Answer from the drawing. Dimensions are ordinates in mm from the lowest x, y and z of the part. Coordinates: 2 decimals unless noted, no trailing zeros. Order: outer loops, then holes, each group sorted by start corner. A loop starts at its lowest first (then second) coordinate and runs counter-clockwise, first axis right, second up. Notation, with made-up numbers: M 58.25,-29.75 L 81.25,-29.75 A15 cw 81.25,-10.75 Z; hole C -18,89.5 d2. An arc over 180 degrees is marked long. Use a Markdown table: item, result.
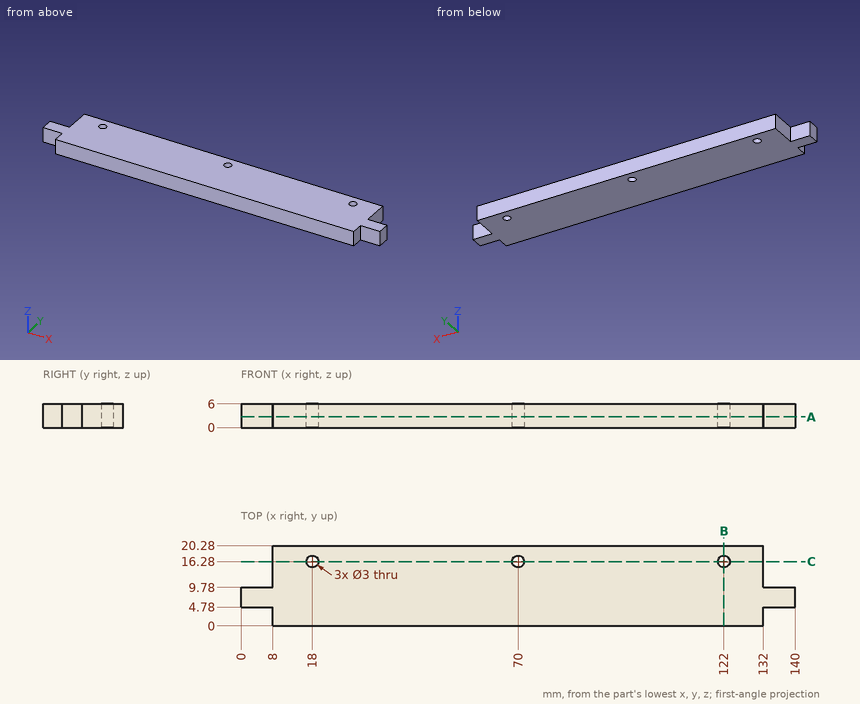
(1) Straight lines are drawn through the part: L1, parallel to Y at x = 18, z = 3.55; L2, parallel to X at y = 15.5, z = 5.05; L3, parallel to X at y = 3.5, z = 2.7. For each, find the intervals that lie inside material, in ascending order.
Conclusion:
| item | result |
|---|---|
| L1 | 0 to 14.78, 17.78 to 20.28 |
| L2 | 8 to 16.72, 19.28 to 68.72, 71.28 to 120.72, 123.28 to 132 |
| L3 | 8 to 132 |
(2) A cutting plane is placed at A-A (z = 2.75). Determine the outline of the cut face in (x, y), then the cut area to 3 significant figures.
Conclusion:
| item | result |
|---|---|
| outline | M 0,4.78 L 8,4.78 L 8,0 L 132,0 L 132,4.78 L 140,4.78 L 140,9.78 L 132,9.78 L 132,20.28 L 8,20.28 L 8,9.78 L 0,9.78 Z; hole C 18,16.28 d3; hole C 70,16.28 d3; hole C 122,16.28 d3 |
| area | 2,570 mm2 |
(3) A cutting plane is placed at B-B (x = 122). Determine the outline of the cut face in (y, z).
Conclusion:
| item | result |
|---|---|
| outline | M 0,0 L 14.78,0 L 14.78,6 L 0,6 Z; M 17.78,0 L 20.28,0 L 20.28,6 L 17.78,6 Z |
(4) A cutting plane is placed at C-C (y = 16.28). Determine the outline of the cut face in (x, z), then the cut area to 3 significant figures.
Conclusion:
| item | result |
|---|---|
| outline | M 8,0 L 16.5,0 L 16.5,6 L 8,6 Z; M 19.5,0 L 68.5,0 L 68.5,6 L 19.5,6 Z; M 71.5,0 L 120.5,0 L 120.5,6 L 71.5,6 Z; M 123.5,0 L 132,0 L 132,6 L 123.5,6 Z |
| area | 690 mm2 |
(5) Given P1, Ø1.8, axis at y = 13, z = 4, coming from the -X side; P2, Ø2.5, axis at x = 70, y = 16.28, coming from the +Z side; P3, Ø1.8, axis at x = 4.5, z = 4, coming from the +Y side, each flat-ended and moving along its own axis, determine where each tip first touches the part or whether it passes through.
Conclusion:
| item | result |
|---|---|
| P1 | x = 8 |
| P2 | through |
| P3 | y = 9.78 |
